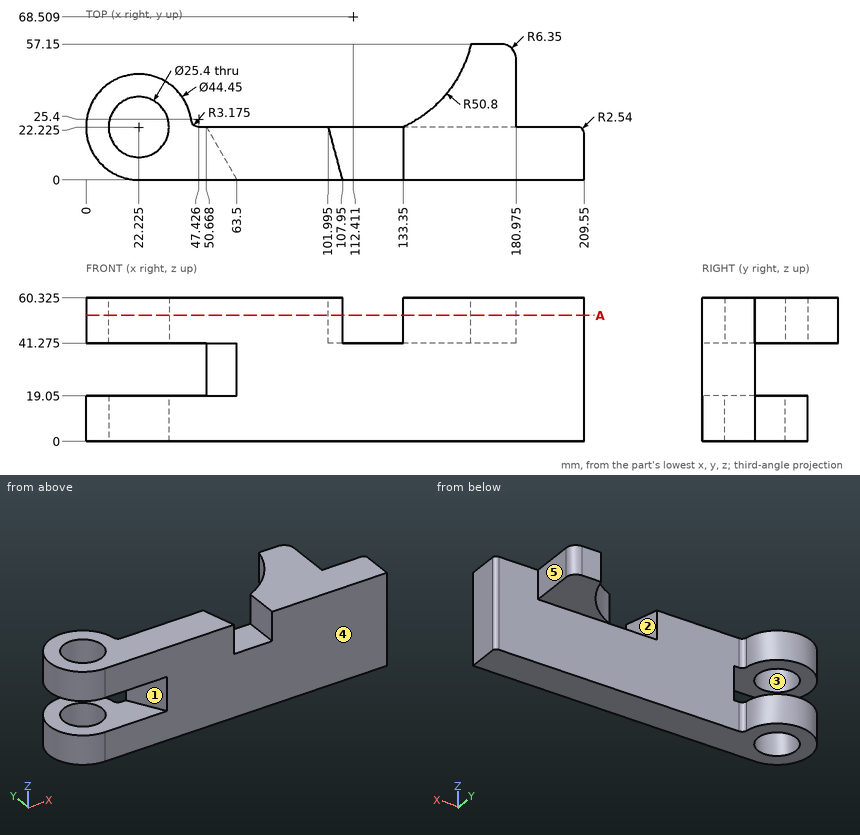
Answer from the drawing. Dimensions are ordinates in mm from the lowest x, y and z of the part. A direction names the side the tool comes from. Give positions to 0.01 mm unless a question says otherwise; leave off trailing zeros. Answer as CSV lines item,"result".
Item 1: Find section A-A on z = 53. State how many separate pieces and enclosed holes the cut face has.
Returned:
separate pieces,"2"
enclosed holes,"1"
Item 2: Each of these flat-tipped pins is pushed along its axis until it touches: pin 1 (18 mm diameter, centred on x = 97.5, z = 24.5, fed in from +Y) (3 decimals); pin 2 (1.5 mm diameter, centred on x = 38.5, y = 34.5, fed in from -Z); pin 3 (17.5 mm diameter, centred on x = 164, y = 37.5, fed in from -Z) (3 decimals); pin 4 (15 mm diameter, centred on y = 13, z = 48.5, fed in from -X). Where does it stop, or does it pass through?
Returned:
pin 1,"stops at y = 22.225"
pin 2,"stops at z = 0"
pin 3,"stops at z = 41.275"
pin 4,"stops at x = 0.07"
Item 3: Consider line 1 (Y direction, x = 201, z = 52.5) (1 decimal); line 2 (X direction, y = 22, z = 28) (1 decimal); line 3 (Y direction, x = 54.5, z = 23) (1 decimal). Determine where each line is inside the solid, lowest interval first. Write a range as [from, to].
Returned:
line 1,"y = [0, 22.2]"
line 2,"x = [50.8, 208.1]"
line 3,"y = [15.6, 22.2]"
Item 4: For the marked faces 1 and 2, determine the directions among +Z, -Z, +X, -X, +Y, -Y from which every point of the face is accessible in a straight line to the end or side of a thin tool.
Returned:
face 1,"-X, -Y"
face 2,"+Z, +Y"
Item 5: Determine the mould class of the marked faces 3, 4 and 5 for opening direction X: +X half, -X half, draft (parallel to the pull), parting line (faces both ways), or undercut.
Returned:
face 3,"undercut"
face 4,"draft"
face 5,"+X half"
